Autodesk Inventor part; units mm, degrees
ref_plane "YZ Plane" through (0, 0, 0) normal (1, 0, 0) x (0, 1, 0)
ref_plane "XZ Plane" through (0, 0, 0) normal (0, 1, 0) x (-1, 0, 0)
ref_plane "XY Plane" through (0, 0, 0) normal (0, 0, 1) x (1, 0, 0)
sketch "Sketch1" plane through (0, 0, 0) normal (0, 0, 1) x (1, 0, 0)
  line L0 (0, 0) -> (0, 25.4)
  line L1 (0, 25.4) -> (25.4, 0)
  line L2 (25.4, 0) -> (0, 0)
  dimension "d0" = 25.4
  dimension "d1" = 25.4
extrude "Extrusion1" add sketch "Sketch1" along normal blind 12.7
sketch "Sketch2" plane through (0, 0, 12.7) normal (0, 0, 1) x (1, 0, 0)
  line L0 (0, 25.4) -> (0, 0)
  line L1 (0, 0) -> (25.4, 0)
  line L2 (25.4, 0) -> (0, 25.4)
  line L3 (1.27, 1.27) -> (22.3339, 1.27)
  line L4 (22.3339, 1.27) -> (1.27, 22.3339)
  line L5 (1.27, 1.27) -> (0, 1.27)
  line L6 (1.27, 22.3339) -> (0, 23.6039)
  line L7 (0, 23.6039) -> (0.898, 24.502)
  line L8 (0, 1.27) -> (0, 23.6039)
  line L9 (0, 23.6039) -> (0, 25.4)
  line L10 (0, 25.4) -> (0.898, 24.502)
  dimension "d4" = 1.27
extrude "Extrusion2" cut sketch "Sketch2" against normal blind 25.4 contours L2 L7 L0 | L6 L4 L3 L5 L0
properties part number "Reinforcer_Front" material "Aluminum 6061"
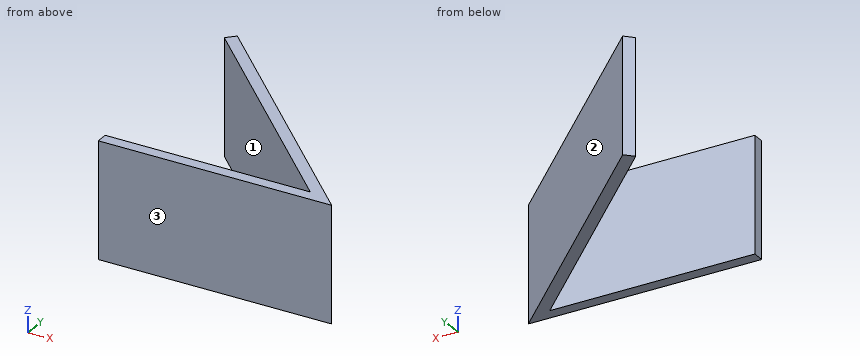
The model under review builds one solid part; all positions refer to its coordinate system, in mm. Face numbers are marked on the shaded views. Round coordinates to 2 decimals unless told otherwise and drop trailing zeros. Write each loop counter-clockwise with the first axis right and the second up, starting at its lowest first coordinate (ties: lowest second). Pieces come first, ordered by that corner, then holes. Notation, with made-up numbers: (-3, 1) - (9, 1) arc R19 ccw to (9, 19) - close; hole circle Ø9 at (33.5, 41.25). An arc over 180 degrees is marked (long way). Use one line per item in the form item = value.
Q1. Consider section B-B (z = 3.5). State the section outline as (x, y) points, and give its area (3 significant figures).
Answer key:
outline = (0, 0) - (25.4, 0) - (0.9, 24.5) - (0, 23.6) - (22.33, 1.27) - (0, 1.27) - close
area = 72.4 mm2
Q2. Insertion check: pin 1 Ø4 at (x, z) = (15, 5.5) entering from +Y; pin 2 Ø3 at (y, z) = (4, 7) entering from +X; pin 3 Ø2 at (y, z) = (10.5, 10) entering from -X; pin 4 Ø3 at (x, y) = (15.5, 7.5) entering from -Z. Each pin has a flat end and moves straight along its axis. Give the tip position at first contact, or say it passes through.
Answer key:
pin_1 = 12.4
pin_2 = 22.9
pin_3 = 12.1
pin_4 = 0
Q3. Draft analysis for pull direction Y (two halves, no side actions). For the marked faces 1, 2 and 3, state which applies: +Y half, -Y half, draft (parallel to the pull), parting line (faces both ways), or undercut.
Answer key:
face_1 = undercut
face_2 = +Y half
face_3 = -Y half
Q4. For line 1 (Y direction, x = 10, z = 11.25); line 2 (Y direction, x = 17.25, z = 3.5); line 3 (X direction, y = 1.5, z = 10), list the stretches that pass through material, from the lowest coordinate up. Write a range as [from, to].
Answer key:
line_1 = [0, 1.27], [13.6, 15.4]
line_2 = [0, 1.27], [6.35, 8.15]
line_3 = [22.1, 23.9]
Q5. Consider section C-C (y = 9). State the section outline as (x, z) points.
Answer key:
outline = (14.6, 0) - (16.4, 0) - (16.4, 12.7) - (14.6, 12.7) - close
Q6. Consider section A-A (x = 19). State the section outline as (y, z) points.
Answer key:
outline = (0, 0) - (1.27, 0) - (1.27, 12.7) - (0, 12.7) - close; (4.6, 0) - (6.4, 0) - (6.4, 12.7) - (4.6, 12.7) - close
